from build123d import *

# Parameters (mm, degrees)
ESBO_O1_R                = 23
ESBO_O1_R_2              = 22
RESSALTO_EXTRUS_O1_DEPTH = 50
ESBO_O2_R                = 7.5
CORTE_EXTRUS_O1_DEPTH    = 50
RESSALTO_EXTRUS_O2_DEPTH = 70
ESBO_O4_R                = 22
CORTE_EXTRUS_O2_DEPTH    = 70
ESBO_O7_R                = 5.5
CORTE_EXTRUS_O4_DEPTH    = 70


with BuildPart() as part:
    # Esboço1 → Ressalto-extrusão1 (new body)
    with BuildSketch(Plane.XY):
        Circle(ESBO_O1_R)
        Circle(ESBO_O1_R_2, mode=Mode.SUBTRACT)
    extrude(amount=RESSALTO_EXTRUS_O1_DEPTH)

    # Esboço2 → Corte-extrusão1 (cut)
    with BuildSketch(Plane(origin=(0, 0, 0), x_dir=(1, 0, 0), z_dir=(0, 1, 0))):
        with Locations(Location((0, -25, 0), (0, 0, 270))):
            Circle(ESBO_O2_R)
    extrude(amount=-CORTE_EXTRUS_O1_DEPTH, mode=Mode.SUBTRACT)

    # Esboço3 → Ressalto-extrusão2 (add)
    with BuildSketch(Plane(origin=(0, 0, 0), x_dir=(1, 0, 0), z_dir=(0, 1, 0))):
        Polygon((0, -7.5), (-12.5, -7.5), (-12.5, -5.5), (12.5, -5.5), (12.5, -7.5), align=None)
        Polygon((0, -42.5), (-12.5, -42.5), (-12.5, -44.5), (12.5, -44.5), (12.5, -42.5), align=None)
    extrude(amount=RESSALTO_EXTRUS_O2_DEPTH)

    # Esboço4 → Corte-extrusão2 (cut)
    with BuildSketch(Plane(origin=(0, 0, 5.5), x_dir=(-1, 0, 0), z_dir=(0, 0, -1))):
        with Locations(Location((0, 0, 0), (0, 0, 180))):
            Circle(ESBO_O4_R)
    extrude(amount=-CORTE_EXTRUS_O2_DEPTH, mode=Mode.SUBTRACT)

    # Esboço7 → Corte-extrusão4 (cut)
    with BuildSketch(Plane(origin=(0, 0, 5.5), x_dir=(-1, 0, 0), z_dir=(0, 0, -1))):
        with Locations((0, 58)):
            Circle(ESBO_O7_R)
    extrude(amount=-CORTE_EXTRUS_O4_DEPTH, mode=Mode.SUBTRACT)


solid = part.part
Build history of the part. All positions in model axes, mm. A direction names the side the tool comes from. Coordinates: 2 decimals unless noted, no trailing zeros. Write each loop counter-clockwise with the first axis right and the second up, starting at its lowest first coordinate (ties: lowest second). Pieces come first, ordered by that corner, then holes.
(1) Drill centre lines: line 1 (Y direction, x = 0, z = 6); line 2 (Z direction, x = 0, y = -22.15); line 3 (Z direction, x = -9, y = 51). Where is each one in solid material? Low to high.
(2) Cut at C-C on y = 0. List the corners of the cut face in (x, z), and give its area (3 significant figures).
(3) Mould opens along X. For faces 1 (the cylindrical face through (0.716, 63.453, 6.486)), 2 (the flat face through (-12.5, 44, 7)), 3 (the flat face through (12.5, 44, 6)), 4 (the flat face through (0, 44, 42.5)) say: pulls with the +X half, pulls with the -X half, needs draft (parallel to the pull), parting line crosses it, or undercut.
(4) Cut at D-D on x = 18.5. List the corners of the cut face in (y, z), and give its area (3 significant figures).
(5) 3-axis set-ups, long thin cutter, end or side, ignore diameter. For faces 5 (the cylindrical face through (-6.654, -21.825, 28.461)), 6 (the flat face through (-12.5, 44, 43)), 7 (the cylindrical face through (-2.994, 22.804, 24.65)), 8 (the flat face through (12.5, 44, 44)): which of +Z, -Z, +X, -X, +Y, -Y reach the whole face in a straight line?
(6) Cut at B-B on x = 0. List the corners of the cut face in (y, z).
(7) Cut at A-A on y = 58. List the corners of the cut face in (x, z).
(8) Pin check, flat tips, straight feed: pin 1 Ø3 at (x, y) = (4.5, 24.5) entering from -Z; pin 2 Ø12 at (x, z) = (-17.5, 30.5) entering from +Y; pin 3 Ø0.6 at (y, z) = (39.5, 6.5) entering from +X. Stop position of each tip, or through.
Working result:
1. line 1: y = -23 to -22, 22 to 52.5, 63.5 to 70
1. line 2: z = 0 to 17.5, 32.5 to 50
1. line 3: z = 5.5 to 7.5, 42.5 to 44.5
2. outline: (-23, 0) - (-22, 0) - (-22, 50) - (-23, 50) - close; (22, 0) - (23, 0) - (23, 50) - (22, 50) - close
2. area: 100 mm2
3. face 1: undercut
3. face 2: pulls with the -X half
3. face 3: pulls with the +X half
3. face 4: needs draft
4. outline: (-13.67, 0) - (-11.91, 0) - (-11.91, 50) - (-13.67, 50) - close; (11.91, 0) - (13.67, 0) - (13.67, 50) - (11.91, 50) - close
4. area: 176 mm2
5. face 5: -Y
5. face 6: +Z, -Z, -X, +Y
5. face 7: none
5. face 8: +Z, -Z, +X, +Y
6. outline: (-23, 0) - (-22, 0) - (-22, 17.5) - (-23, 17.5) - close; (-23, 32.5) - (-22, 32.5) - (-22, 50) - (-23, 50) - close; (22, 0) - (23, 0) - (23, 5.5) - (52.5, 5.5) - (52.5, 7.5) - (23, 7.5) - (23, 42.5) - (52.5, 42.5) - (52.5, 44.5) - (23, 44.5) - (23, 50) - (22, 50) - close; (63.5, 5.5) - (70, 5.5) - (70, 7.5) - (63.5, 7.5) - close; (63.5, 42.5) - (70, 42.5) - (70, 44.5) - (63.5, 44.5) - close
7. outline: (-12.5, 5.5) - (-5.5, 5.5) - (-5.5, 7.5) - (-12.5, 7.5) - close; (-12.5, 42.5) - (-5.5, 42.5) - (-5.5, 44.5) - (-12.5, 44.5) - close; (5.5, 5.5) - (12.5, 5.5) - (12.5, 7.5) - (5.5, 7.5) - close; (5.5, 42.5) - (12.5, 42.5) - (12.5, 44.5) - (5.5, 44.5) - close
8. pin 1: stops at z = 5.5
8. pin 2: stops at y = 19.92
8. pin 3: stops at x = 12.5
